from build123d import *

# Parameters (mm, degrees)
F0_W     = 57.15
F0_H     = 44.45
F1_DEPTH = 38.1
F2_W     = 57.15
F2_H     = 38.1
F3_DEPTH = 19.05
F4_R     = 5.08
F5_W     = 31.75
F5_H     = 12.7
F6_DEPTH = 19.051
F8_DEPTH = 6.351


with BuildPart() as f1:
    # F0 (on Front) → F1 (new body)
    with BuildSketch(Plane.XZ):
        with Locations((28.575, 22.225)):
            Rectangle(F0_W, F0_H)
    extrude(amount=F1_DEPTH)

    # F2 (on face) → F3 (cut)
    with BuildSketch(Plane.XZ.offset(38.1)):
        with Locations((28.575, 25.4)):
            Rectangle(F2_W, F2_H)
    extrude(amount=-F3_DEPTH, mode=Mode.SUBTRACT)

    # F4
    f4_edges = [f1.edges().sort_by_distance(p)[0] for p in [
        (0, -38.1, 3.175),
        (57.15, -38.1, 3.175),
    ]]
    fillet(f4_edges, radius=F4_R)

    # F5 (on face) → F6 (cut, through all)
    with BuildSketch(Plane.XZ.offset(19.05)):
        with BuildLine():
            Line((12.7, 31.75), (12.7, 38.1659469176))
            ThreePointArc((12.7, 38.1659469176), (8.1632404269, 36.2867595731), (6.2840530824, 31.75))
            Line((6.2840530824, 31.75), (12.7, 31.75))
        make_face()
        with BuildLine():
            ThreePointArc((19.1159469176, 31.75), (17.2367595731, 36.2867595731), (12.7, 38.1659469176))
            Line((12.7, 38.1659469176), (12.7, 31.75))
            Line((12.7, 31.75), (19.1159469176, 31.75))
        make_face()
        with BuildLine():
            Line((12.7, 25.3340530824), (12.7, 31.75))
            Line((12.7, 31.75), (6.2840530824, 31.75))
            ThreePointArc((6.2840530824, 31.75), (8.1632404269, 27.2132404269), (12.7, 25.3340530824))
        make_face()
        with BuildLine():
            Line((19.1159469176, 31.75), (12.7, 31.75))
            Line((12.7, 31.75), (12.7, 25.3340530824))
            ThreePointArc((12.7, 25.3340530824), (17.2367595731, 27.2132404269), (19.1159469176, 31.75))
        make_face()
        with BuildLine():
            Line((12.7, 43.9009574959), (12.7, 44.45))
            Line((12.7, 44.45), (0, 44.45))
            Line((0, 44.45), (0, 31.75))
            ThreePointArc((0, 31.75), (3.9117156386, 40.3739372872), (12.7, 43.9009574959))
        make_face()
        with BuildLine():
            Line((25.4, 44.45), (12.7, 44.45))
            Line((12.7, 44.45), (12.7, 43.9009574959))
            ThreePointArc((12.7, 43.9009574959), (21.4882843614, 40.3739372872), (25.4, 31.75))
            Line((25.4, 31.75), (25.4, 44.45))
        make_face()
        with BuildLine():
            Line((57.15, 31.75), (25.4, 31.75))
            ThreePointArc((25.4, 31.75), (29.6571125542, 17.2352579477), (40.1600599289, 6.35))
            Line((40.1600599289, 6.35), (57.15, 6.35))
            Line((57.15, 6.35), (57.15, 31.75))
        make_face()
        with Locations((41.275, 38.1)):
            Rectangle(F5_W, F5_H)
    extrude(amount=-F6_DEPTH, mode=Mode.SUBTRACT)

    # F7 (on face) → F8 (cut, through all)
    with BuildSketch(Plane.XY.offset(6.35)):
        with BuildLine():
            Line((1.9419096436, -33.02), (8.2180903564, -33.02))
            ThreePointArc((8.2180903564, -33.02), (5.08, -29.8819096436), (1.9419096436, -33.02))
        make_face()
        with BuildLine():
            ThreePointArc((1.9419096436, -33.02), (5.08, -36.1580903564), (8.2180903564, -33.02))
            Line((8.2180903564, -33.02), (1.9419096436, -33.02))
        make_face()
        with BuildLine():
            Line((45.4800299644, -33.02), (51.8300299644, -33.02))
            ThreePointArc((51.8300299644, -33.02), (48.6550299644, -29.845), (45.4800299644, -33.02))
        make_face()
        with BuildLine():
            ThreePointArc((45.4800299644, -33.02), (48.6550299644, -36.195), (51.8300299644, -33.02))
            Line((51.8300299644, -33.02), (45.4800299644, -33.02))
        make_face()
        with BuildLine():
            Line((45.4016557758, -9.525), (51.9084041531, -9.525))
            ThreePointArc((51.9084041531, -9.525), (48.6550299644, -6.2716258113), (45.4016557758, -9.525))
        make_face()
        with BuildLine():
            ThreePointArc((45.4016557758, -9.525), (48.6550299644, -12.7783741887), (51.9084041531, -9.525))
            Line((51.9084041531, -9.525), (45.4016557758, -9.525))
        make_face()
    extrude(amount=-F8_DEPTH, mode=Mode.SUBTRACT)


solid = f1.part
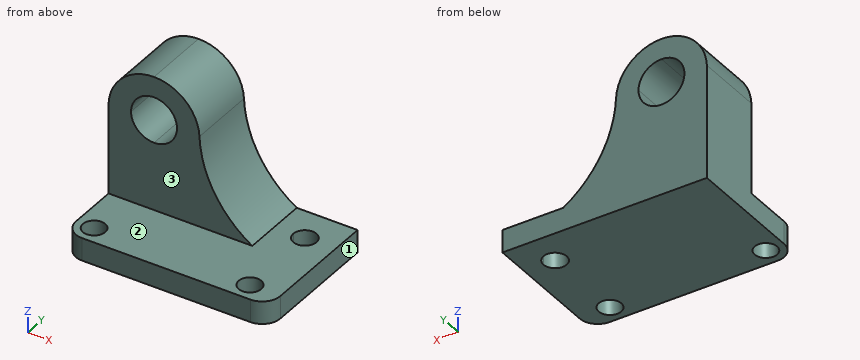
Input: part model. Units: mm. Frame: model coordinates. Face numbers are marked on the shaded views. A direction names the side the tool comes from. Give positions to 0.01 mm unless a question says otherwise; leave off trailing zeros. Order: outer loops, then holes, each group sorted by start corner. A loop starts at its lowest first (then second) coordinate and runs counter-clockwise, first axis right, second up.
Q1. Set-up query: the marked faces 1, 2 and 3. Return all of +Z, -Z, +X, -X, +Y, -Y with unobstructed straight access to the full face (end or side cutting, diameter ignored); none if empty.
Checked values:
face 1: +Z, -Z, +X, +Y, -Y
face 2: +Z, +X, -Y
face 3: +Z, +X, -X, -Y
Q2. Contact query for flat-ended pins moving along their axis: pin 1 Ø1.5 at (x, z) = (26, 9) entering from -Y; pin 2 Ø3 at (y, z) = (-10, 34) entering from +X; pin 3 Ø1.5 at (x, y) = (49, -19) entering from +Z. Output: stop coordinate, or through.
Checked values:
pin 1: stops at y = -19.05
pin 2: stops at x = 25.34
pin 3: stops at z = 6.35
Q3. Ray query, probe 1 along X at (y, z) = (-33.02, 4); probe 2 along Y at (x, z) = (5.08, 3); probe 3 along Y at (x, z) = (36.5, 7). Return the intervals inside material, ascending.
Checked values:
probe 1: x = 0 to 1.94, 8.22 to 45.48, 51.83 to 57.15
probe 2: y = -38.1 to -36.16, -29.88 to 0
probe 3: y = -19.05 to 0
Q4. Section A-A on z = 4.5. Output: boundary loops of the cut face in (x, y) (3 decimals), and give its area (3 significant figures).
Checked values:
outline: (0, -33.02) arc R5.08 ccw to (5.08, -38.1) - (52.07, -38.1) arc R5.08 ccw to (57.15, -33.02) - (57.15, 0) - (0, 0) - close; hole circle Ø6.276 at (5.08, -33.02); hole circle Ø6.507 at (48.655, -9.525); hole circle Ø6.35 at (48.655, -33.02)
area: 2,070 mm2
Q5. Section D-D on x = 28. Output: boundary loops of the cut face in (y, z).
Checked values:
outline: (-38.1, 0) - (0, 0) - (0, 20.51) - (-19.05, 20.51) - (-19.05, 6.35) - (-38.1, 6.35) - close
Q6. Section C-C on y = -31.5. Output: boundary loops of the cut face in (x, z), and give its area (3 significant figures).
Checked values:
outline: (0, 0) - (2.33, 0) - (2.33, 6.35) - (0, 6.35) - close; (7.83, 0) - (45.87, 0) - (45.87, 6.35) - (7.83, 6.35) - close; (51.44, 0) - (57.15, 0) - (57.15, 6.35) - (51.44, 6.35) - close
area: 293 mm2
Q7. Section B-B on y = -13.5. Output: boundary loops of the cut face in (x, z), and give its area (3 significant figures).
Checked values:
outline: (0, 0) - (57.15, 0) - (57.15, 6.35) - (40.16, 6.35) arc R31.67 cw to (25.4, 31.75) arc R12.71 ccw to (0, 31.75) - close; hole circle Ø12.83 at (12.7, 31.75)
area: 1,230 mm2
